Check sheet for the modelled part. Datum: model origin and axes. Units: mm. A direction names the side the tool comes from. Give positions to 0.01 mm unless a question says otherwise; leave off trailing zeros. Write each loop counter-clockwise with the first axis right and the second up, starting at its lowest first coordinate (ties: lowest second). Pieces come first, ordered by that corner, then holes. Notation, with made-up numbers: (-24.5, 83) -> (2.5, 83) arc R14 cw to (2.5, 104) -> close; hole circle Ø10 at (4, 78.5). An arc over 180 degrees is marked (long way). Answer as a JSON object with one key per item and string values.
from build123d import *

# Parameters (mm, degrees)
SKETCH1_W           = 9
SKETCH1_H           = 75
BOSS_EXTRUDE1_DEPTH = 26
RIB3_REACH          = 65.738
SKETCH3_WALL_W      = 172.022520638
SKETCH3_WALL_H      = 6


with BuildPart() as part:
    # Sketch1 → Boss-Extrude1 (new, symmetric)
    with BuildSketch(Plane(origin=(0, 0, 0), x_dir=(1, 0, 0), z_dir=(0, 1, 0))):
        Rectangle(SKETCH1_W, SKETCH1_H)
        with BuildLine():
            Line((4.5, 4.5), (4.5, -4.5))
            Line((4.5, -4.5), (21.944512863, -4.5))
            ThreePointArc((21.944512863, -4.5), (21.5, 0), (21.944512863, 4.5))
            Line((21.944512863, 4.5), (4.5, 4.5))
        make_face()
        with BuildLine():
            Line((44.5, -15), (44.5, -23))
            ThreePointArc((44.5, -23), (21.5, 0), (44.5, 23))
            Line((44.5, 23), (44.5, 15))
            ThreePointArc((44.5, 15), (29.5, 0), (44.5, -15))
        make_face()
    extrude(amount=BOSS_EXTRUDE1_DEPTH, both=True)

    # Sketch3 wall → Rib3 (add, up to next)
    with BuildSketch(Plane(origin=(24.5, 0, 30.25), x_dir=(-0.940136065162, 0, 0.340799323621), z_dir=(0.340799323621, 0, 0.940136065162)), mode=Mode.PRIVATE) as rib3_sk1:
        Rectangle(SKETCH3_WALL_W, SKETCH3_WALL_H)
    rib3_tool1 = extrude(rib3_sk1.sketch, amount=-RIB3_REACH, mode=Mode.PRIVATE) - part.part
    add(rib3_tool1.solids().sort_by_distance((24.5, 0, 30.25))[0])


solid = part.part
1. Sectioned sample at C-C, the plane y = 10.5. Enter the section's corners in (x, z).
Determined:
{"outline": "(-4.5, -37.5) -> (4.5, -37.5) -> (4.5, -4.5) -> (21.94, -4.5) arc R23 ccw to (44.5, -23) -> (44.5, -15) arc R15 cw to (44.5, 15) -> (44.5, 23) arc R23 ccw to (21.94, 4.5) -> (4.5, 4.5) -> (4.5, 37.5) -> (-4.5, 37.5) -> close"}
2. Sectioned sample at B-B, the plane x = 34. Enter the section's corners in (y, z).
Determined:
{"outline": "(-26, -20.46) -> (26, -20.46) -> (26, -10.71) -> (-26, -10.71) -> close; (-26, 10.71) -> (26, 10.71) -> (26, 20.46) -> (3, 20.46) -> (3, 26.81) -> (-3, 26.81) -> (-3, 20.46) -> (-26, 20.46) -> close"}
3. Sectioned sample at A-A, the plane z = -11. Enter the section's corners in (x, y).
Determined:
{"outline": "(-4.5, -26) -> (4.5, -26) -> (4.5, 26) -> (-4.5, 26) -> close; (24.3, -26) -> (34.3, -26) -> (34.3, 26) -> (24.3, 26) -> close"}
4. Sectioned sample at D-D, the plane x = 12.5. Enter the section's corners in (y, z), plus the area to 3 significant figures.
Determined:
{"outline": "(-26, -4.5) -> (26, -4.5) -> (26, 4.5) -> (3, 4.5) -> (3, 34.6) -> (-3, 34.6) -> (-3, 4.5) -> (-26, 4.5) -> close", "area": "649 mm^2"}
5. Access from +Z, -Z, +X, -X, +Y, -Y to the whole of each face (thin tool, end or side, straight path). Record for faces 1 (the face through (14, 26, -1)), 2 (the face through (16, 3, 21)), 3 (the face through (4.5, -14, 21)), 4 (the face through (13, 0, -4.5)), 5 (the face through (14, -26, -1)).
Determined:
{"face 1": "+Z, -Z, +X, -X, +Y", "face 2": "+Z, +Y", "face 3": "+Z, -Y", "face 4": "-Z, +Y, -Y", "face 5": "+Z, -Z, +X, -X, -Y"}
6. Mould release check, pull along X, two halves, no side actions. Record for faces 6 (the face through (0, 0, 37.5)), 7 (the face through (30.086, -14.339, 17.923)), 8 (the face through (29.504, 0.364, -0.33)): released by +X, released by -X, zero draft, split by the parting line, or undercut.
Determined:
{"face 6": "zero draft", "face 7": "undercut", "face 8": "released by +X"}
7. Scan lines: L1, parallel to Z at x = 19, y = 20.5; L2, parallel to X at y = 4.5, z = 11.5. Record each from-to range of solid material in increasing order. Write a range as [from, to].
Determined:
{"L1": "[-4.5, 4.5]", "L2": "[-4.5, 4.5], [24.58, 34.87]"}
8. Go/stop test with flat-tipped pins: P1, Ø8.5, axis at x = 10, y = 16, coming from the +Z side; P2, Ø12, axis at x = 36.5, y = 0.5, coming from the +Z side (3 decimals); P3, Ø3, axis at x = 14, y = -14.5, coming from the -Z side; P4, Ø1, axis at x = 31.5, z = -4.5, coming from the -Y side. Record where each tip stops, or that it passes through.
Determined:
{"P1": "z = 4.5", "P2": "z = 28.075", "P3": "z = -4.5", "P4": "through"}
